Design review of the part built by this model. Coordinates are the model's own, in mm. A direction names the side the tool comes from. Round coordinates to 2 decimals unless told otherwise and drop trailing zeros. Write each loop counter-clockwise with the first axis right and the second up, starting at its lowest first coordinate (ties: lowest second). Pieces come first, ordered by that corner, then holes.
from build123d import *

# Parameters (mm, degrees)
BOX016_W          = 2
BOX016_H          = 10
BOX016_DEPTH      = 10
FILLET008_R       = 0.95
BOX017_W          = 3
BOX017_H          = 5
BOX017_DEPTH      = 10
CYLINDER011_R     = 2
CYLINDER011_DEPTH = 10
CYLINDER010_R     = 1
CYLINDER010_DEPTH = 10
CYLINDER005_R     = 1
CYLINDER005_DEPTH = 10
CYLINDER004_R     = 1
CYLINDER004_DEPTH = 10
CYLINDER009_R     = 1.2
CYLINDER009_DEPTH = 0.1
CYLINDER008_R     = 1.2
CYLINDER008_DEPTH = 0.1
BOX011_W          = 9
BOX011_H          = 2
BOX011_DEPTH      = 0.3
BOX012_W          = 9
BOX012_H          = 2
BOX012_DEPTH      = 0.3
CYLINDER006_R     = 1.5
CYLINDER006_DEPTH = 10
CYLINDER007_R     = 1.5
CYLINDER007_DEPTH = 10
BOX010_W          = 8
BOX010_H          = 16
BOX010_DEPTH      = 1.2
CYLINDER003_R     = 2.5
CYLINDER003_DEPTH = 0.3
CYLINDER002_R     = 2.5
CYLINDER002_DEPTH = 0.3
BOX009_W          = 9
BOX009_H          = 16
BOX009_DEPTH      = 0.3
BOX003_W          = 133
BOX003_H          = 63
BOX003_DEPTH      = 0.5
FILLET004_R       = 1
BOX007_W          = 4
BOX007_H          = 63
BOX007_DEPTH      = 1
FILLET006_R       = 1
BOX018_W          = 3
BOX018_H          = 5
BOX018_DEPTH      = 10
FILLET009_R       = 1.49
BOX006_W          = 8
BOX006_H          = 63
BOX006_DEPTH      = 1
FILLET007_R       = 1


with BuildPart() as fillet008:
    # Box016 → Box016 (new body)
    with BuildSketch(Plane(origin=(4, 28.5, 0), x_dir=(1, 0, 0), z_dir=(0, 0, 1))):
        with Locations((1, 5)):
            Rectangle(BOX016_W, BOX016_H)
    extrude(amount=BOX016_DEPTH)

    # Fillet008
    fillet008_edges = [fillet008.edges().sort_by_distance(p)[0] for p in [
        (4, 28.5, 5),
        (4, 38.5, 5),
        (6, 28.5, 5),
        (6, 38.5, 5),
    ]]
    fillet(fillet008_edges, radius=FILLET008_R)


with BuildPart() as cubo011:
    # Box017 → Box017 (new body)
    with BuildSketch(Plane(origin=(3.5, 21, 0), x_dir=(1, 0, 0), z_dir=(0, 0, 1))):
        with Locations((1.5, 2.5)):
            Rectangle(BOX017_W, BOX017_H)
    extrude(amount=BOX017_DEPTH)


with BuildPart() as cilindro011:
    # Cylinder011 → Cylinder011 (new body)
    with BuildSketch(Plane(origin=(5.5, 44, 0), x_dir=(1, 0, 0), z_dir=(0, 0, 1))):
        Circle(CYLINDER011_R)
    extrude(amount=CYLINDER011_DEPTH)


with BuildPart() as cilindro010:
    # Cylinder010 → Cylinder010 (new body)
    with BuildSketch(Plane(origin=(5.5, 50, 0), x_dir=(1, 0, 0), z_dir=(0, 0, 1))):
        Circle(CYLINDER010_R)
    extrude(amount=CYLINDER010_DEPTH)


with BuildPart() as cilindro005:
    # Cylinder005 → Cylinder005 (new body)
    with BuildSketch(Plane(origin=(38.5, 11, 1), x_dir=(1, 0, 0), z_dir=(0, 0, 1))):
        Circle(CYLINDER005_R)
    extrude(amount=CYLINDER005_DEPTH)


with BuildPart() as cilindro004:
    # Cylinder004 → Cylinder004 (new body)
    with BuildSketch(Plane(origin=(38.5, 27, 1), x_dir=(1, 0, 0), z_dir=(0, 0, 1))):
        Circle(CYLINDER004_R)
    extrude(amount=CYLINDER004_DEPTH)


with BuildPart() as cilindro009:
    # Cylinder009 → Cylinder009 (new body)
    with BuildSketch(Plane(origin=(38.5, 27, 1), x_dir=(1, 0, 0), z_dir=(0, 0, 1))):
        Circle(CYLINDER009_R)
    extrude(amount=CYLINDER009_DEPTH)


with BuildPart() as cilindro008:
    # Cylinder008 → Cylinder008 (new body)
    with BuildSketch(Plane(origin=(38.5, 11, 1), x_dir=(1, 0, 0), z_dir=(0, 0, 1))):
        Circle(CYLINDER008_R)
    extrude(amount=CYLINDER008_DEPTH)


with BuildPart() as cubo008:
    # Box011 → Box011 (new body)
    with BuildSketch(Plane(origin=(34, 11, 5.5), x_dir=(1, 0, 0), z_dir=(0, 0, 1))):
        with Locations((4.5, 1)):
            Rectangle(BOX011_W, BOX011_H)
    extrude(amount=BOX011_DEPTH)


with BuildPart() as cubo009:
    # Box012 → Box012 (new body)
    with BuildSketch(Plane(origin=(34, 25, 5.5), x_dir=(1, 0, 0), z_dir=(0, 0, 1))):
        with Locations((4.5, 1)):
            Rectangle(BOX012_W, BOX012_H)
    extrude(amount=BOX012_DEPTH)


with BuildPart() as cilindro006:
    # Cylinder006 → Cylinder006 (new body)
    with BuildSketch(Plane(origin=(38.5, 11, 1), x_dir=(1, 0, 0), z_dir=(0, 0, 1))):
        Circle(CYLINDER006_R)
    extrude(amount=CYLINDER006_DEPTH)


with BuildPart() as cilindro007:
    # Cylinder007 → Cylinder007 (new body)
    with BuildSketch(Plane(origin=(38.5, 27, 1), x_dir=(1, 0, 0), z_dir=(0, 0, 1))):
        Circle(CYLINDER007_R)
    extrude(amount=CYLINDER007_DEPTH)


with BuildPart() as cut008:
    # Box010 → Box010 (new body)
    with BuildSketch(Plane(origin=(34.5, 11, 5), x_dir=(1, 0, 0), z_dir=(0, 0, 1))):
        with Locations((4, 8)):
            Rectangle(BOX010_W, BOX010_H)
    extrude(amount=BOX010_DEPTH)

    # Cut001: cut Cilindro004
    add(cilindro004.part, mode=Mode.SUBTRACT)

    # Cut002: cut Cilindro005
    add(cilindro005.part, mode=Mode.SUBTRACT)

    # Cut007: cut Cilindro007
    add(cilindro007.part, mode=Mode.SUBTRACT)

    # Cut008: cut Cilindro006
    add(cilindro006.part, mode=Mode.SUBTRACT)


with BuildPart() as cilindro003:
    # Cylinder003 → Cylinder003 (new body)
    with BuildSketch(Plane(origin=(38.5, 27, 1), x_dir=(1, 0, 0), z_dir=(0, 0, 1))):
        Circle(CYLINDER003_R)
    extrude(amount=CYLINDER003_DEPTH)


with BuildPart() as cilindro002:
    # Cylinder002 → Cylinder002 (new body)
    with BuildSketch(Plane(origin=(38.5, 11, 1), x_dir=(1, 0, 0), z_dir=(0, 0, 1))):
        Circle(CYLINDER002_R)
    extrude(amount=CYLINDER002_DEPTH)


with BuildPart() as dont_show:
    # Box009 → Box009 (new body)
    with BuildSketch(Plane(origin=(34, 11, 1), x_dir=(1, 0, 0), z_dir=(0, 0, 1))):
        with Locations((4.5, 8)):
            Rectangle(BOX009_W, BOX009_H)
    extrude(amount=BOX009_DEPTH)

    # Fusion001: union Cilindro003, Cilindro002
    add(cilindro003.part)
    add(cilindro002.part)


with BuildPart() as dont_show_1:
    # Fusion001 placement: moved
    add(dont_show.part.moved(Location((0, 0, 4.4))))

    # Cut003: cut Cilindro005
    add(cilindro005.part, mode=Mode.SUBTRACT)

    # Cut004: cut Cilindro004
    add(cilindro004.part, mode=Mode.SUBTRACT)


with BuildPart() as dont_show_2:
    # Cut004 placement: moved
    add(dont_show_1.part.moved(Location((0, 0, 0.4))))

    # Fusion002: union Cut008
    add(cut008.part)


with BuildPart() as cut022:
    # Box003 → Box003 (new body)
    with BuildSketch(Plane(origin=(2, 2, 5.5), x_dir=(1, 0, 0), z_dir=(0, 0, 1))):
        with Locations((66.5, 31.5)):
            Rectangle(BOX003_W, BOX003_H)
    extrude(amount=BOX003_DEPTH)

    # Fillet004
    fillet004_edges = [cut022.edges().sort_by_distance(p)[0] for p in [
        (2, 2, 5.75),
        (2, 65, 5.75),
        (135, 2, 5.75),
        (135, 65, 5.75),
    ]]
    fillet(fillet004_edges, radius=FILLET004_R)

    # Cut009: cut Dont show
    add(dont_show_2.part, mode=Mode.SUBTRACT)

    # Fusion003: union Cubo008, Cubo009
    add(cubo008.part)
    add(cubo009.part)

    # Cut010: cut Cilindro008
    add(cilindro008.part, mode=Mode.SUBTRACT)

    # Cut011: cut Cilindro009
    add(cilindro009.part, mode=Mode.SUBTRACT)

    # Cut012: cut Cilindro004
    add(cilindro004.part, mode=Mode.SUBTRACT)

    # Cut013: cut Cilindro005
    add(cilindro005.part, mode=Mode.SUBTRACT)

    # Cut017: cut Cilindro010
    add(cilindro010.part, mode=Mode.SUBTRACT)

    # Cut019: cut Cilindro011
    add(cilindro011.part, mode=Mode.SUBTRACT)

    # Cut020: cut Cubo011
    add(cubo011.part, mode=Mode.SUBTRACT)

    # Cut022: cut Fillet008
    add(fillet008.part, mode=Mode.SUBTRACT)


with BuildPart() as bottom:
    # Box007 → Box007 (new body)
    with BuildSketch(Plane(origin=(131, 2, 6), x_dir=(1, 0, 0), z_dir=(0, 0, 1))):
        with Locations((2, 31.5)):
            Rectangle(BOX007_W, BOX007_H)
    extrude(amount=BOX007_DEPTH)

    # Fillet006
    fillet006_edges = [bottom.edges().sort_by_distance(p)[0] for p in [
        (135, 2, 6.5),
        (135, 65, 6.5),
    ]]
    fillet(fillet006_edges, radius=FILLET006_R)


with BuildPart() as fillet009:
    # Box018 → Box018 (new body)
    with BuildSketch(Plane(origin=(3.5, 21, 0), x_dir=(1, 0, 0), z_dir=(0, 0, 1))):
        with Locations((1.5, 2.5)):
            Rectangle(BOX018_W, BOX018_H)
    extrude(amount=BOX018_DEPTH)

    # Fillet009
    fillet009_edges = [fillet009.edges().sort_by_distance(p)[0] for p in [
        (3.5, 21, 5),
        (3.5, 26, 5),
        (6.5, 21, 5),
        (6.5, 26, 5),
    ]]
    fillet(fillet009_edges, radius=FILLET009_R)


with BuildPart() as fusion004:
    # Box006 → Box006 (new body)
    with BuildSketch(Plane(origin=(2, 2, 6), x_dir=(1, 0, 0), z_dir=(0, 0, 1))):
        with Locations((4, 31.5)):
            Rectangle(BOX006_W, BOX006_H)
    extrude(amount=BOX006_DEPTH)

    # Fillet007
    fillet007_edges = [fusion004.edges().sort_by_distance(p)[0] for p in [
        (2, 2, 6.5),
        (2, 65, 6.5),
    ]]
    fillet(fillet007_edges, radius=FILLET007_R)

    # Cut015: cut Fillet008
    add(fillet008.part, mode=Mode.SUBTRACT)

    # Cut018: cut Cilindro010
    add(cilindro010.part, mode=Mode.SUBTRACT)

    # Cut021: cut Fillet009
    add(fillet009.part, mode=Mode.SUBTRACT)

    # Cut023: cut Cilindro011
    add(cilindro011.part, mode=Mode.SUBTRACT)

    # Fusion004: union Cut022, Bottom
    add(cut022.part)
    add(bottom.part)


solid = fusion004.part
1) Add section C-C on y = 54.5. State the section outline as (x, z) points, and give its area (3 significant figures).
2) The part is to be moulded in two halves that separate along X. For faces 1 (the face through (70, 34, 6)), 2 (the face through (68, 34, 5.5)), say which applies: pulls with the +X half, pulls with the -X half, needs draft (parallel to the pull), parting line crosses it, or undercut.
3) For line 1 along Y through (x, z) = (38.5, 5.6); line 2 along X through (y, z) = (32, 6.45); line 3 along X through (y, z) = (50, 6.55), list the stretches that pass through material, from the lowest coordinate up.
4) For P1, Ø1, axis at x = 96, y = 41, coming from the +Z side; P2, Ø2.5, axis at x = 38.5, y = 11, coming from the +Z side, all flat-tipped, find the tip position at first contact; note any pin that passes through.
5) For faces 3 (the face through (5.066, 42.048, 6.24)), 4 (the face through (37, 12, 5.8)), list the 3-axis set-ups (+Z, -Z, +X, -X, +Y, -Y) from which the entire face can be reached by the end or side of a thin tool; tool diameter is ignored.
6) Add section B-B on y = 44. State the section outline as (x, z) points.
7) Add section A-A on z = 6.6. Count the separate pieces of the cut face and the enclosed holes in it, and give its area (3 significant figures).
8) Add section D-D on x = 70. State the section outline as (y, z) points.
Computed:
1. outline: (2, 5.5) - (135, 5.5) - (135, 7) - (131, 7) - (131, 6) - (10, 6) - (10, 7) - (2, 7) - close
1. area: 78.5 mm2
2. face 1: undercut
2. face 2: needs draft
3. line 1: y = 2 to 10, 12 to 13, 25 to 26, 28 to 65
3. line 2: x = 2 to 4, 6 to 10, 131 to 135
3. line 3: x = 2 to 4.5, 6.5 to 10, 131 to 135
4. P1: stops at z = 6
4. P2: stops at z = 5.8
5. face 3: +Z, -Z
5. face 4: +Z
6. outline: (2, 5.5) - (3.5, 5.5) - (3.5, 7) - (2, 7) - close; (7.5, 5.5) - (135, 5.5) - (135, 7) - (131, 7) - (131, 6) - (10, 6) - (10, 7) - (7.5, 7) - close
7. separate pieces: 2
7. enclosed holes: 4
7. area: 707 mm2
8. outline: (2, 5.5) - (65, 5.5) - (65, 6) - (2, 6) - close
